Autodesk Inventor part; units mm, degrees
ref_plane "YZ Plane" through (0, 0, 0) normal (1, 0, 0) x (0, 1, 0)
ref_plane "XZ Plane" through (0, 0, 0) normal (0, 1, 0) x (-1, 0, 0)
ref_plane "XY Plane" through (0, 0, 0) normal (0, 0, 1) x (1, 0, 0)
sketch "スケッチ1" plane through (0, 0, 0) normal (0, 0, 1) x (1, 0, 0)
  circle A0 centre (0, 0) radius 75
  dimension "d0" = 150
extrude "押し出し1" add sketch "スケッチ1" along normal blind 10
sketch "スケッチ2" plane through (0, 0, 10) normal (0, 0, 1) x (1, 0, 0)
  circle A0 centre (0, 0) radius 77
  dimension "d3" = 154
extrude "押し出し2" add sketch "スケッチ2" along normal blind 1
sketch "スケッチ3" plane through (0, 0, 0) normal (0, 0, -1) x (-1, 0, 0)
  circle A0 centre (0, 0) radius 77
  dimension "d6" = 154
extrude "押し出し3" add sketch "スケッチ3" along normal blind 1
sketch "スケッチ4" plane through (0, 0, 11) normal (0, 0, 1) x (1, 0, 0)
  circle A0 centre (0, 0) radius 4
  dimension "d9" = 8
extrude "押し出し4" cut sketch "スケッチ4" against normal blind 12
properties part number "射出_type0" material "アセタール樹脂、白"
For this review, take the finished solid that the model builds, in its own axes (mm). A direction names the side the tool comes from. Round coordinates to 2 decimals unless told otherwise and drop trailing zeros. Write each loop counter-clockwise with the first axis right and the second up, starting at its lowest first coordinate (ties: lowest second). Pieces come first, ordered by that corner, then holes. Notation, with made-up numbers: (-5.5, -23.5) -> (47.5, -23.5) arc R11 ccw to (47.5, -4.5) -> close; hole circle Ø9 at (39, -33.5). An arc over 180 degrees is marked (long way). Put each result on its own line as item: value.
Q1. Consider section C-C on z = 3.5. State the section outline as (x, y) points.
Determined:
outline: circle Ø150 at (0, 0); hole circle Ø8 at (0, 0)
Q2. Machinability: for faces 1 (the cylindrical face through (-61.105, 46.853, 10.493)), 2 (the flat face through (-17, -74, 0)), which of the approach directions +Z, -Z, +X, -X, +Y, -Y give a long, thin tool a straight path to every point of the face, cutting with its end or side? Answer none if there is none.
Determined:
face 1: +Z, -Z
face 2: none
Q3. Clearance check with flat-ended pins moving along their axes: pin 1 Ø3 at (y, z) = (8, 0.5) entering from +X; pin 2 Ø2 at (x, z) = (-5, 7) entering from +Y; pin 3 Ø6 at (x, z) = (-51.5, 5.5) entering from +Y. State where each tip first meets the part, or that it passes through.
Determined:
pin 1: stops at x = 76.72
pin 2: stops at y = 74.89
pin 3: stops at y = 57.21
Q4. To check wall thickness, follow L1, parallel to Y at x = 0, z = 6; L2, parallel to Y at x = -3, z = 1.5; L3, parallel to Y at x = -25.5, z = 4.25. State the ranges of each line that lie inside material, in increasing order. Write a range as [from, to].
Determined:
L1: y = [-75, -4], [4, 75]
L2: y = [-74.94, -2.65], [2.65, 74.94]
L3: y = [-70.53, 70.53]
Q5. Consider section D-D on x = -44.5. State the section outline as (y, z) points.
Determined:
outline: (-62.84, -1) -> (62.84, -1) -> (62.84, 0) -> (60.37, 0) -> (60.37, 10) -> (62.84, 10) -> (62.84, 11) -> (-62.84, 11) -> (-62.84, 10) -> (-60.37, 10) -> (-60.37, 0) -> (-62.84, 0) -> close
Q6. Consider section A-A on y = 0. State the section outline as (x, z) points, and give its area (3 significant figures).
Determined:
outline: (-77, -1) -> (-4, -1) -> (-4, 11) -> (-77, 11) -> (-77, 10) -> (-75, 10) -> (-75, 0) -> (-77, 0) -> close; (4, -1) -> (77, -1) -> (77, 0) -> (75, 0) -> (75, 10) -> (77, 10) -> (77, 11) -> (4, 11) -> close
area: 1,710 mm^2
Q7. The part is to be moulded in two halves that separate along Z. For faces 3 (the cylindrical face through (-9.764, -74.362, 4.93)), 4 (the flat face through (-1, -16, 11)), 5 (the cylindrical face through (-0.867, -3.905, 5.084)), 6 (the flat face through (1, -16, -1)), say which applies: released by +Z, released by -Z, zero draft, split by the parting line, or undercut.
Determined:
face 3: undercut
face 4: released by +Z
face 5: zero draft
face 6: released by -Z
